Here's the drawing with two shaded views (mm, measured from the low corner). I have some questions. A direction names the side the tool comes from. Give positions to 0.01 mm unless a question says otherwise; leave off trailing zeros. Loops run counter-clockwise (first coordinate to the right, second up) from the corner with the lowest first, then second, coordinate; pieces in that order, holes last. Notation, with made-up numbers: (-26, 0) - (-4, 0) arc R22 ccw to (-4, 28) - close; hole circle Ø7 at (-17.5, -39). An arc over 180 degrees is marked (long way). Use one line per item in the form item = value.
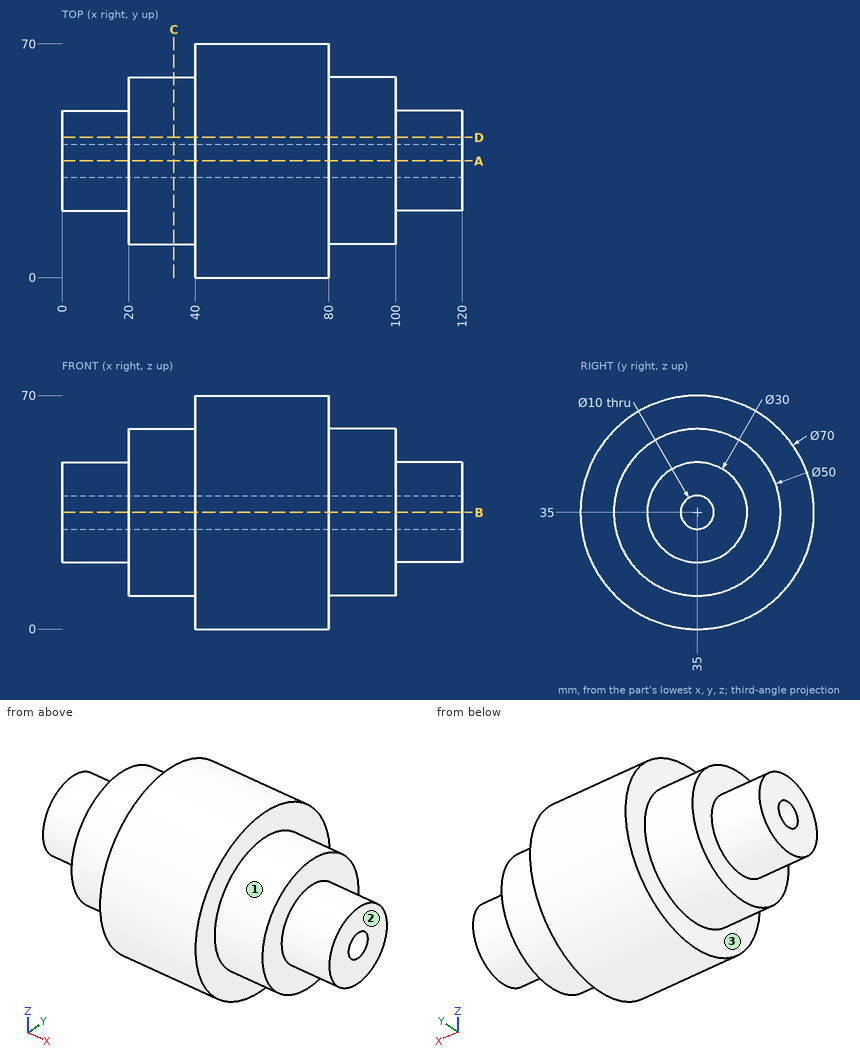
(1) If we section it at D-D (y = 42): List the corners of the cut face in (x, z) for me, plus the area to 3 significant figures.
Geometry says:
outline = (0, 21.73) - (20, 21.73) - (20, 11) - (40, 11) - (40, 0.71) - (80, 0.71) - (80, 11) - (100, 11) - (100, 21.73) - (120, 21.73) - (120, 48.27) - (100, 48.27) - (100, 59) - (80, 59) - (80, 69.29) - (40, 69.29) - (40, 59) - (20, 59) - (20, 48.27) - (0, 48.27) - close
area = 5,720 mm²
(2) If I drill on probe 1 along Z at (x, y) = (90.5, 35); probe 2 along Z at (x, y) = (63, 35), over which ranges is the centre line in solid material (lowest first)?
Geometry says:
probe_1 = 10 to 30, 40 to 60
probe_2 = 0 to 30, 40 to 70
(3) For the marked faces 1, 2 and 3, which set-ups out of +Z, -Z, +X, -X, +Y, -Y let a thin tool reach every point of the face, with its end or its side?
Geometry says:
face_1 = +X
face_2 = +Z, -Z, +X, +Y, -Y
face_3 = -X
(4) If we section it at A-A (y = 35): List the corners of the cut face in (x, z) for me, plus the area to 3 significant figures.
Geometry says:
outline = (0, 20) - (20, 20) - (20, 10) - (40, 10) - (40, 0) - (80, 0) - (80, 10) - (100, 10) - (100, 20) - (120, 20) - (120, 30) - (0, 30) - close; (0, 40) - (120, 40) - (120, 50) - (100, 50) - (100, 60) - (80, 60) - (80, 70) - (40, 70) - (40, 60) - (20, 60) - (20, 50) - (0, 50) - close
area = 4,800 mm²
(5) If we section it at C-C (x = 33.5): List the corners of the cut face in (y, z) for me, plus the area to 3 significant figures.
Geometry says:
outline = circle Ø50 at (35, 35); hole circle Ø10 at (35, 35)
area = 1,880 mm²
(6) For P1, Ø15, axis at y = 33.5, z = 35, coming from the +X side; P2, Ø10, axis at x = 21.5, y = 40.5, coming from the +Z side (3 decimals); P3, Ø3, axis at y = 28.5, z = 11.5, coming from the -X side; P4, Ø6, axis at x = 90.5, z = 15, coming from the +Y side, each with a flat end and sliding along its axis, tell me the tip position at first contact or that it passes through.
Geometry says:
P1 = 120
P2 = 59.995
P3 = 20
P4 = 53.33
